Autodesk Inventor part; units mm, degrees
ref_plane "YZ Plane" through (0, 0, 0) normal (1, 0, 0) x (0, 1, 0)
ref_plane "XZ Plane" through (0, 0, 0) normal (0, 1, 0) x (-1, 0, 0)
ref_plane "XY Plane" through (0, 0, 0) normal (0, 0, 1) x (1, 0, 0)
sketch "Skizze1" plane through (0, 0, 0) normal (0, 0, 1) x (1, 0, 0)
  line L0 (-45, 12) -> (45, 12)
  line L1 (45, 12) -> (45, -12)
  line L2 (45, -12) -> (-45, -12)
  line L3 (-45, -12) -> (-45, 12)
  line L4 (-45, 12) -> (45, -12) construction
  line L5 (45, 12) -> (-45, -12) construction
  point P0 (0, 0)
  dimension "d0" = 24
  dimension "d1" = 90
extrude "Extrusion1" add sketch "Skizze1" along normal blind 1
sketch "Skizze4" plane through (0, 0, 1) normal (0, 0, 1) x (1, 0, 0)
  line L0 (15, -9.1) -> (-15, -9.1) construction
  line L1 (15, -8.2) -> (-15, -8.2)
  line L2 (-15, -10) -> (15, -10)
  arc A0 (15, -10) -> (15, -8.2) centre (15, -9.1) ccw
  arc A1 (-15, -8.2) -> (-15, -10) centre (-15, -9.1) ccw
  line L3 (0, 17) -> (0, -18)
  line L4 (-45, -12) -> (45, -12)
  point P0 (0, 0)
  point P1 (0, -9.1)
  dimension "d25" = 1.8
  dimension "d26" = 30
  dimension "d27" = 2
extrude "Extrusion2" cut sketch "Skizze4" against normal through all
sketch "Skizze2" plane through (0, 0, 1) normal (0, 0, 1) x (1, 0, 0)
  line L0 (31, 9) -> (-31, 9) construction
  line L1 (45, 12) -> (-45, 12)
  line L2 (0, 20.4) -> (0, -17.4)
  line L3 (-45, -12) -> (45, -12)
  dimension "d5" = 62
  dimension "d48" = 21
hole "Bohrung1" at (-31, 9, 1) at (31, 9, 1) direction (0, 0, -1) diameter 3.1 end through all
sketch "Skizze5" plane through (0, 0, 1) normal (0, 0, 1) x (1, 0, 0)
  line L0 (-45, -12) -> (45, -12)
  line L1 (0, 17.4) -> (0, -20.4)
  point P0 (0, 0)
  point P1 (22.05, -5.3)
  point P2 (-22.05, -5.3)
  dimension "d30" = 6.7
  dimension "d31" = 44.1
hole "Bohrung3" at (22.05, -5.3, 1) at (-22.05, -5.3, 1) direction (0, 0, -1) diameter 2.1 end through all
sketch "Skizze7" plane through (0, 0, 1) normal (0, 0, 1) x (1, 0, 0)
  line L0 (0, 20.4) -> (0, -17.4)
  line L1 (-45, -12) -> (45, -12)
  line L2 (-22, 12) -> (-14, 12)
  line L3 (-14, 12) -> (-14, 5)
  line L4 (-14, 5) -> (-22, 5)
  line L5 (-22, 5) -> (-22, 12)
  line L6 (-18, 5) -> (-18, 12) construction
  line L7 (45, 12) -> (-45, 12) construction
  point P0 (0, 0)
  dimension "d49" = 18
  dimension "d50" = 17
  dimension "d51" = 8
extrude "Extrusion4" cut sketch "Skizze7" against normal through all
chamfer "Fase1" distance 1 angle 45 2 edges at (-22, 5, 0.5) (-14, 5, 0.5)
properties part number "Ballsensorplatine" material "Phenolharz"
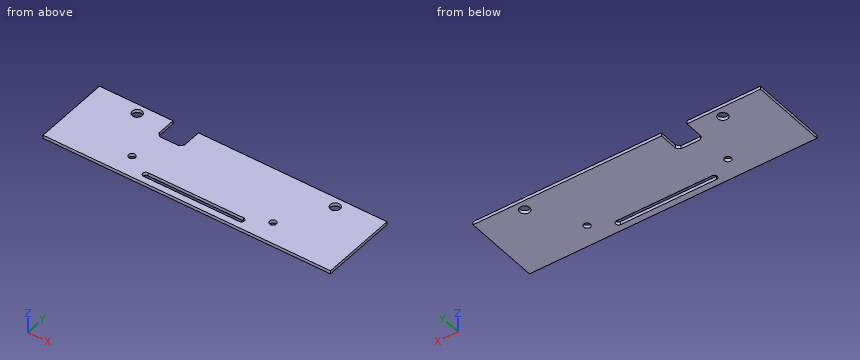
Geometry check sheet. Reference: the model listing, model coordinates, mm. Round coordinates to 2 decimals unless told otherwise and drop trailing zeros. Order: outer loops, then holes, each group sorted by start corner. A loop starts at its lowest first (then second) coordinate and runs counter-clockwise, first axis right, second up. Notation, with made-up numbers: M 2,48.5 L 57,48.5 A25 ccw 57,77.5 Z; hole C 89.5,29.5 d5. An arc over 180 degrees is marked long. Answer in a Markdown table with one row per item.
(1) Sectioned sample at A-A, the plane x = -31. Record the cut outline in (y, z), and give its area (3 significant figures).
Responses:
| item | result |
|---|---|
| outline | M -12,0 L 7.45,0 L 7.45,1 L -12,1 Z; M 10.55,0 L 12,0 L 12,1 L 10.55,1 Z |
| area | 20.9 mm² |
(2) Scan lines: probe 1 along X at (y, z) = (9, 0.6); probe 2 along Y at (x, z) = (-31, 0.4); probe 3 along Y at (x, z) = (-2.5, 0.55). Record each from-to range of solid material in increasing order. Write a range as from..to.
Responses:
| item | result |
|---|---|
| probe 1 | x = -45..-32.55, -29.45..-22, -14..29.45, 32.55..45 |
| probe 2 | y = -12..7.45, 10.55..12 |
| probe 3 | y = -12..-10, -8.2..12 |
(3) Sectioned sample at C-C, the plane z = 0.55. Record the cut outline in (x, y), and give its area (3 significant figures).
Responses:
| item | result |
|---|---|
| outline | M -45,-12 L 45,-12 L 45,12 L -14,12 L -14,6 L -15,5 L -21,5 L -22,6 L -22,12 L -45,12 Z; hole C -31,9 d3.1; hole C -22.05,-5.3 d2.1; hole M -15,-10 L 15,-10 A0.9 ccw 15,-8.2 L -15,-8.2 A0.9 ccw Z; hole C 22.05,-5.3 d2.1; hole C 31,9 d3.1 |
| area | 2,030 mm² |
(4) Sectioned sample at D-D, the plane y = -5.3. Record the cut outline in (x, z), and give its area (3 significant figures).
Responses:
| item | result |
|---|---|
| outline | M -45,0 L -23.1,0 L -23.1,1 L -45,1 Z; M -21,0 L 21,0 L 21,1 L -21,1 Z; M 23.1,0 L 45,0 L 45,1 L 23.1,1 Z |
| area | 85.8 mm² |
(5) Sectioned sample at B-B, the plane y = 9. Record the cut outline in (x, z).
Responses:
| item | result |
|---|---|
| outline | M -45,0 L -32.55,0 L -32.55,1 L -45,1 Z; M -29.45,0 L -22,0 L -22,1 L -29.45,1 Z; M -14,0 L 29.45,0 L 29.45,1 L -14,1 Z; M 32.55,0 L 45,0 L 45,1 L 32.55,1 Z |
